Verification items for the finished model (mm, model axes). A direction names the side the tool comes from. Round coordinates to 2 decimals unless told otherwise and drop trailing zeros. Write each loop counter-clockwise with the first axis right and the second up, starting at its lowest first coordinate (ties: lowest second). Pieces come first, ordered by that corner, then holes. Notation, with made-up numbers: (88, 10) -> (120, 10) arc R23 ccw to (120, 32) -> close; hole circle Ø11 at (34.25, -26). An arc over 180 degrees is marked (long way). Use CSV: the item, a comma, the result in double quotes.
```python
from build123d import *

# Parameters (mm, degrees)
SKETCH1_R           = 49
BOSS_EXTRUDE1_DEPTH = 4
BOSS_EXTRUDE2_DEPTH = 20
BOSS_EXTRUDE3_DEPTH = 13.5
SKETCH3_4_R         = 6
BOSS_EXTRUDE4_DEPTH = 13.5
CUT_EXTRUDE5_DEPTH  = 5.5
CUT_EXTRUDE6_DEPTH  = 9
SKETCH11_W          = 7
SKETCH11_H          = 7
BOSS_EXTRUDE5_DEPTH = 10
CUT_EXTRUDE9_REACH  = 112.656
SKETCH12_W          = 3
SKETCH12_H          = 6
FILLET1_R           = 2
CUT_EXTRUDE10_REACH = 97.458
SKETCH13_R          = 1.27
CUT_EXTRUDE11_DEPTH = 95
CUT_EXTRUDE12_DEPTH = 2
CUT_EXTRUDE13_DEPTH = 2
CUT_EXTRUDE14_REACH = 97.458
SKETCH17_R          = 1.09
CUT_EXTRUDE15_REACH = 106.754
SKETCH18_R          = 2.01


with BuildPart() as part:
    # Sketch1 → Boss-Extrude1 (new body)
    with BuildSketch(Plane(origin=(0, 0, 0), x_dir=(1, 0, 0), z_dir=(0, 1, 0))):
        with Locations(Location((0, 0, 0), (0, 0, 270))):
            Circle(SKETCH1_R)
    extrude(amount=BOSS_EXTRUDE1_DEPTH)

    # Sketch3 → Boss-Extrude2 (add)
    with BuildSketch(Plane.XY.offset(4)):
        with BuildLine():
            Line((-30.347886599, 11), (-30.347886599, 4))
            Line((-30.347886599, 4), (-18.049754955, 4))
            ThreePointArc((-18.049754955, 4), (-22.391739007, 19.253033546), (-32.784586802, 31.232039038))
            ThreePointArc((-32.784586802, 31.232039038), (-36.760767526, 57.926722426), (-10.066084138, 61.902903149))
            ThreePointArc((-10.066084138, 61.902903149), (11.703451168, 36.427560581), (20.150880429, 4))
            Line((20.150880429, 4), (28.656645727, 4))
            Line((28.656645727, 4), (27.702300884, 11))
            ThreePointArc((27.702300884, 11), (16.110760067, 42.048857672), (-7.685218322, 65.117164801))
            ThreePointArc((-7.685218322, 65.117164801), (-39.975029178, 60.307588242), (-35.165452618, 28.017777386))
            ThreePointArc((-35.165452618, 28.017777386), (-31.452519142, 19.87808091), (-30.347886599, 11))
        make_face()
    extrude(amount=BOSS_EXTRUDE2_DEPTH)

    # Sketch3<3> → Boss-Extrude3 (add)
    with BuildSketch(Plane.XY.offset(4)):
        with BuildLine():
            ThreePointArc((-32.784586802, 31.232039038), (-22.391739007, 19.253033546), (-18.049754955, 4))
            Line((-18.049754955, 4), (20.150880429, 4))
            ThreePointArc((20.150880429, 4), (11.703451168, 36.427560581), (-10.066084138, 61.902903149))
            ThreePointArc((-10.066084138, 61.902903149), (-36.760767526, 57.926722426), (-32.784586802, 31.232039038))
        make_face()
        Polygon((14.142135624, 25.142135624), (0, 11), (-28.496403282, 39.496403282), (-14.354267658, 53.638538906), align=None, mode=Mode.SUBTRACT)
    extrude(amount=BOSS_EXTRUDE3_DEPTH)

    # Sketch3<4> → Boss-Extrude4 (add)
    # profile 1 of 2: a face of its own
    with BuildSketch(Plane.XY.offset(4)):
        Polygon((-28.496403282, 39.496403282), (-14.354267658, 53.638538906), (14.142135624, 25.142135624), (0, 11), align=None)
        with Locations((-14.297699116, 39.439834739)):
            Circle(SKETCH3_4_R, mode=Mode.SUBTRACT)
    # profile 2 of 2: a face of its own
    with BuildSketch(Plane.XY.offset(4)):
        with Locations((-14.297699116, 39.439834739)):
            Circle(SKETCH3_4_R)
    extrude(amount=BOSS_EXTRUDE4_DEPTH)

    # Sketch5 → Cut-Extrude5 (cut)
    with BuildSketch(Plane.XY.offset(17.5)):
        Polygon((15.321499667, 20.547344219), (-24.135058723, 60.003902609), (-38.277194347, 45.861766985), (1.179364043, 6.405208595), align=None)
    extrude(amount=-CUT_EXTRUDE5_DEPTH, mode=Mode.SUBTRACT)

    # Sketch8 → Cut-Extrude6 (cut)
    with BuildSketch(Plane.XY.offset(12)):
        Polygon((-18.761047186, 54.629891072), (-32.90318281, 40.487755448), (-4.194647494, 11.779220132), (9.94748813, 25.921355756), align=None)
    extrude(amount=-CUT_EXTRUDE6_DEPTH, mode=Mode.SUBTRACT)

    # Sketch11 → Boss-Extrude5 (add)
    with BuildSketch(Plane(origin=(0, 4, 0), x_dir=(1, 0, 0), z_dir=(0, 1, 0))):
        with Locations((25.156645727, 3.5)):
            Rectangle(SKETCH11_W, SKETCH11_H)
    extrude(amount=BOSS_EXTRUDE5_DEPTH)

    # Sketch12 → Cut-Extrude9 (cut, up to next)
    with BuildSketch(Plane.ZY.offset(-21.656645727), mode=Mode.PRIVATE) as cut_extrude9_sk1:
        with Locations((-3.5, 9)):
            Rectangle(SKETCH12_W, SKETCH12_H)
    cut_extrude9_tool1 = extrude(cut_extrude9_sk1.sketch, amount=-CUT_EXTRUDE9_REACH, mode=Mode.PRIVATE) & part.part
    add(cut_extrude9_tool1.solids().sort_by_distance((21.656646, 9, -3.5))[0], mode=Mode.SUBTRACT)

    # Fillet1
    fillet1_edges = [part.edges().sort_by_distance(p)[0] for p in [
        (25.156645727, 14, 0),
        (25.156645727, 14, -7),
    ]]
    fillet(fillet1_edges, radius=FILLET1_R)

    # Sketch13 → Cut-Extrude10 (cut, up to next)
    with BuildSketch(Plane(origin=(0, 4, 0), x_dir=(1, 0, 0), z_dir=(0, 1, 0)), mode=Mode.PRIVATE) as cut_extrude10_sk1:
        with Locations(Location((0, 0, 0), (0, 0, 270))):
            Circle(SKETCH13_R)
    cut_extrude10_tool1 = extrude(cut_extrude10_sk1.sketch, amount=-CUT_EXTRUDE10_REACH, mode=Mode.PRIVATE) & part.part
    add(cut_extrude10_tool1.solids().sort_by_distance((0, 4, 0))[0], mode=Mode.SUBTRACT)

    # Sketch14 → Cut-Extrude11 (cut, symmetric)
    with BuildSketch(Plane.XY.offset(17.5)):
        Polygon((-49, 1.5), (50.231696903, 1.5), (50.231696903, 0), (-50.303866734, 0), (-50.303866734, 1.5), align=None)
    extrude(amount=CUT_EXTRUDE11_DEPTH, both=True, mode=Mode.SUBTRACT)

    # Sketch16 → Cut-Extrude12 (cut)
    with BuildSketch(Plane.XY.offset(12)):
        Polygon((3.583527099, 19.557394725), (2.876420318, 18.850287944), (8.250431855, 13.476276407), (8.957538636, 14.183383188), align=None)
        Polygon((8.250431855, 13.476276407), (2.876420318, 18.850287944), (2.169313537, 18.143181163), (7.543325074, 12.769169626), align=None)
    extrude(amount=-CUT_EXTRUDE12_DEPTH, mode=Mode.SUBTRACT)

    # Sketch16<3> → Cut-Extrude13 (cut)
    with BuildSketch(Plane.XY.offset(12)):
        Polygon((-25.832114998, 47.55882326), (-31.206126535, 52.932834797), (-31.913233317, 52.225728016), (-26.53922178, 46.851716479), align=None)
        Polygon((-30.499019754, 53.639941578), (-31.206126535, 52.932834797), (-25.832114998, 47.55882326), (-25.125008217, 48.265930041), align=None)
    extrude(amount=-CUT_EXTRUDE13_DEPTH, mode=Mode.SUBTRACT)

    # Sketch17 → Cut-Extrude14 (cut, up to next)
    with BuildSketch(Plane(origin=(0, 4, 0), x_dir=(1, 0, 0), z_dir=(0, 1, 0)), mode=Mode.PRIVATE) as cut_extrude14_sk1:
        with Locations(Location((8.18, 0, 0), (0, 0, 270))):
            Circle(SKETCH17_R)
    cut_extrude14_tool1 = extrude(cut_extrude14_sk1.sketch, amount=-CUT_EXTRUDE14_REACH, mode=Mode.PRIVATE) & part.part
    # Sketch17 → Cut-Extrude14 (cut, up to next)
    with BuildSketch(Plane(origin=(0, 4, 0), x_dir=(1, 0, 0), z_dir=(0, 1, 0)), mode=Mode.PRIVATE) as cut_extrude14_sk2:
        with Locations(Location((-8.18, 0, 0), (0, 0, 270))):
            Circle(SKETCH17_R)
    cut_extrude14_tool2 = extrude(cut_extrude14_sk2.sketch, amount=-CUT_EXTRUDE14_REACH, mode=Mode.PRIVATE) & part.part
    # Sketch17 → Cut-Extrude14 (cut, up to next)
    with BuildSketch(Plane(origin=(0, 4, 0), x_dir=(1, 0, 0), z_dir=(0, 1, 0)), mode=Mode.PRIVATE) as cut_extrude14_sk3:
        with Locations(Location((0, 8.18, 0), (0, 0, 270))):
            Circle(SKETCH17_R)
    cut_extrude14_tool3 = extrude(cut_extrude14_sk3.sketch, amount=-CUT_EXTRUDE14_REACH, mode=Mode.PRIVATE) & part.part
    add(cut_extrude14_tool1.solids().sort_by_distance((8.18, 4, 0))[0], mode=Mode.SUBTRACT)
    add(cut_extrude14_tool2.solids().sort_by_distance((-8.18, 4, 0))[0], mode=Mode.SUBTRACT)
    add(cut_extrude14_tool3.solids().sort_by_distance((0, 4, -8.18))[0], mode=Mode.SUBTRACT)

    # Sketch18 → Cut-Extrude15 (cut, up to next)
    with BuildSketch(Plane.XY.offset(12), mode=Mode.PRIVATE) as cut_extrude15_sk1:
        with Locations((2.593577605, 12.062062844)):
            Circle(SKETCH18_R)
    cut_extrude15_tool1 = extrude(cut_extrude15_sk1.sketch, amount=-CUT_EXTRUDE15_REACH, mode=Mode.PRIVATE) & part.part
    # Sketch18 → Cut-Extrude15 (cut, up to next)
    with BuildSketch(Plane.XY.offset(12), mode=Mode.PRIVATE) as cut_extrude15_sk2:
        with Locations((9.664645417, 19.133130656)):
            Circle(SKETCH18_R)
    cut_extrude15_tool2 = extrude(cut_extrude15_sk2.sketch, amount=-CUT_EXTRUDE15_REACH, mode=Mode.PRIVATE) & part.part
    # Sketch18 → Cut-Extrude15 (cut, up to next)
    with BuildSketch(Plane.XY.offset(12), mode=Mode.PRIVATE) as cut_extrude15_sk3:
        with Locations((-32.620340098, 47.275980548)):
            Circle(SKETCH18_R)
    cut_extrude15_tool3 = extrude(cut_extrude15_sk3.sketch, amount=-CUT_EXTRUDE15_REACH, mode=Mode.PRIVATE) & part.part
    # Sketch18 → Cut-Extrude15 (cut, up to next)
    with BuildSketch(Plane.XY.offset(12), mode=Mode.PRIVATE) as cut_extrude15_sk4:
        with Locations((-25.549272286, 54.347048359)):
            Circle(SKETCH18_R)
    cut_extrude15_tool4 = extrude(cut_extrude15_sk4.sketch, amount=-CUT_EXTRUDE15_REACH, mode=Mode.PRIVATE) & part.part
    add(cut_extrude15_tool1.solids().sort_by_distance((2.593578, 12.062063, 12))[0], mode=Mode.SUBTRACT)
    add(cut_extrude15_tool2.solids().sort_by_distance((9.664645, 19.133131, 12))[0], mode=Mode.SUBTRACT)
    add(cut_extrude15_tool3.solids().sort_by_distance((-32.62034, 47.275981, 12))[0], mode=Mode.SUBTRACT)
    add(cut_extrude15_tool4.solids().sort_by_distance((-25.549272, 54.347048, 12))[0], mode=Mode.SUBTRACT)


solid = part.part
```
Q1. Section check C-C (z = 29). Record the cut outline in (x, y), plus the area to 3 significant figures.
Filled in:
outline,"(-39.5, 1.5) -> (39.5, 1.5) -> (39.5, 4) -> (-39.5, 4) -> close"
area,"197 mm²"
Q2. Mould release check, pull along Z, two halves, no side actions. Record for faces 5 (the flat face through (-4, 42, 17.5)), 6 (the flat face through (8.151, 13.377, 14.636)), 7 (the flat face through (25, 6, -4)), 8 (the cylindrical face through (14.718, 2.732, 46.737)): released by +Z, released by -Z, zero draft, split by the parting line, or undercut.
Filled in:
face 5,"released by +Z"
face 6,"zero draft"
face 7,"undercut"
face 8,"split by the parting line"
Q3. Section check A-A (y = 34). Record the cut outline in (x, z).
Filled in:
outline,"(-40.79, 4) -> (-26.42, 4) -> (-26.42, 17.5) -> (-35.79, 17.5) -> (-35.79, 24) -> (-40.79, 24) -> close; (1.87, 4) -> (20.69, 4) -> (20.69, 24) -> (12.91, 24) -> (12.91, 17.5) -> (1.87, 17.5) -> close"
Q4. Go/stop test with flat-tipped pins: P1, Ø13, axis at x = 12, y = 22, coming from the +Z side; P2, Ø5.5, axis at y = 8.5, z = -2, coming from the -X side; P3, Ø1, axis at x = -5.5, z = -35, coming from the +Y side; P4, Ø2.5, axis at x = -25.55, y = 54.35, coming from the -Z side. Record where each tip stops, or that it passes through.
Filled in:
P1,"z = 24"
P2,"x = 21.66"
P3,"y = 4"
P4,"through"
Q5. Access from +Z, -Z, +X, -X, +Y, -Y to the whole of each face (thin tool, end or side, straight path). Record for faces 1 (the flat face through (25, 14, -4)), 2 (the cylindrical face through (2.16, 10.1, 8.06)), 3 (the flat face through (-30.348, 8, 14)), 4 (the flat face through (6.31, 16.83, 11.01)).
Filled in:
face 1,"-Z, +X, -X, +Y"
face 2,"+Z, -Z"
face 3,"+Z, -Z, -X"
face 4,"+Z"
Q6. Material ranges on L1, parallel to X at y = 2, z = 0; L2, parallel to X at y = 49, z = 8.5; L3, parallel to Z at x = -39, y = 57, recorded low to high.
Filled in:
L1,"-49 to -9.27, -7.09 to -1.27, 1.27 to 7.09, 9.27 to 49"
L2,"-44.38 to -33.65, -31.59 to -24.39, -13.13 to 10.97"
L3,"4 to 24"
Q7. Section check B-B (x = 40.5). Record the cut outline in (y, z), plus the area to 3 significant figures.
Filled in:
outline,"(1.5, -27.58) -> (4, -27.58) -> (4, 27.58) -> (1.5, 27.58) -> close"
area,"138 mm²"
